Input: part model. Units: mm. Frame: model coordinates. Face numbers are marked on the shaded views. A direction names the side the tool comes from. Round coordinates to 2 decimals unless told otherwise and drop trailing zeros. Loops run counter-clockwise (first coordinate to the right, second up) from the corner with the lowest first, then second, coordinate; pieces in that order, holes last.
(1) Draft query along X for the marked faces 1, 2 and 3. Return one class per face: released by +X, released by -X, zero draft, split by the parting line, or undercut.
(2) Cut plane B-B, the plane y = -4.5. Output: boundary loops of the cut face in (x, z).
(3) Access query for the marked faces 4 and 5. Directions: +Z, -Z, +X, -X, +Y, -Y. A direction counts if a zero-diameter tool reaches every point of the face in a straight line with its end or side. Return the directions, or none.
(4) First-contact query: pin 1 Ø3 at (x, y) = (3, -5.5) entering from +Z; pin 2 Ø2 at (y, z) = (-7, -10) entering from +X; pin 3 Ø10 at (x, y) = (-11, -1) entering from -Z; pin 4 Ø13.5 at (x, z) = (0, 0) entering from +Y. Flat tips, straight axial feed; report the tip coordinate or a pass-through.
(5) Line query: line 1 (X direction, y = -6, z = 0); line 2 (Z direction, x = 0, y = -4); line 3 (X direction, y = 5, z = 0). Output: solid intervals per line, ascending.
(6) Cut plane A-A, the plane z = 0. Output: boundary loops of the cut face in (x, y), and give its area (3 significant figures).
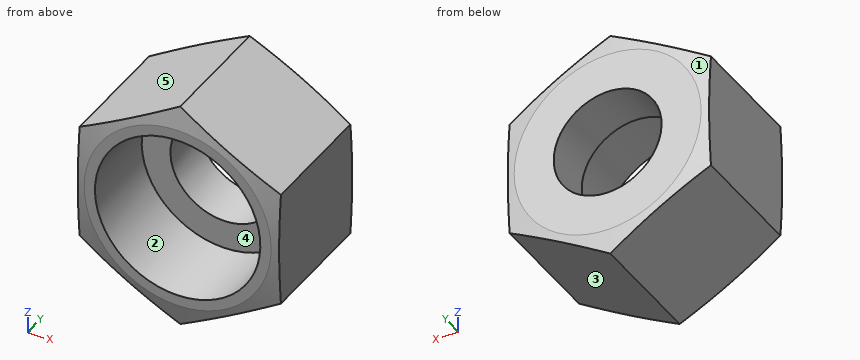
Solid Edge part; units mm, degrees
sketch "Sketch1" plane through (0, 0, 0) normal (0, -1, 0) x (1, 0, 0)
  line L0 (0, -16.1658) -> (14, -8.0829)
  line L1 (14, -8.0829) -> (14, 8.0829)
  line L2 (14, 8.0829) -> (0, 16.1658)
  line L3 (0, 16.1658) -> (-14, 8.0829)
  line L4 (-14, 8.0829) -> (-14, -8.0829)
  line L5 (-14, -8.0829) -> (0, -16.1658)
extrude "Protrusion1" add sketch "Sketch1" along normal mid plane 18
sketch "Sketch2" plane through (0, 0, 0) normal (1, 0, 0) x (0, 1, 0)
  line L0 (9, -13) -> (7.6451, -19.7097)
revolve "RevolvedCutout1" cut sketch "Sketch2" angle 360 about axis through (0, -63.5, 0) along (0, 1, 0) material side at (0, 8.3716, -16.3647)
mirror "Mirror1" about plane through (0, 0, 0) normal (0, -1, 0) of "RevolvedCutout1"
sketch "Sketch3" plane through (0, 0, 0) normal (1, 0, 0) x (0, 1, 0)
  line L0 (-9, -11.5) -> (2.2546, -11.5)
  line L1 (2.2546, -11.5) -> (2.2546, -7.5)
  line L2 (2.2546, -7.5) -> (9, -7.5)
revolve "RevolvedCutout3" cut sketch "Sketch3" angle 360 about axis through (0, -63.5, 0) along (0, 1, 0) material side at (0, -3.3727, -11.45)
Reported:
1. face 1: split by the parting line
1. face 2: undercut
1. face 3: released by +X
2. outline: (-14, -8.08) - (0, -16.17) - (14, -8.08) - (14, 8.08) - (0, 16.17) - (-14, 8.08) - close; hole circle Ø23 at (0, 0)
3. face 4: -Y
3. face 5: +Z, -X, +Y, -Y
4. pin 1: stops at z = 15.3
4. pin 2: stops at x = 12.41
4. pin 3: stops at z = -12.7
4. pin 4: passes through
5. line 1: x = -14 to -11.5, 11.5 to 14
5. line 2: z = -16.17 to -11.5, 11.5 to 16.17
5. line 3: x = -14 to -7.5, 7.5 to 14
6. outline: (-14, -8.8) - (-13, -9) - (-11.5, -9) - (-11.5, 2.25) - (-7.5, 2.25) - (-7.5, 9) - (-13, 9) - (-14, 8.8) - close; (7.5, 2.25) - (11.5, 2.25) - (11.5, -9) - (13, -9) - (14, -8.8) - (14, 8.8) - (13, 9) - (7.5, 9) - close
6. area: 144 mm2
